Part model, mm, in its own coordinate system. Coordinates: 2 decimals unless noted, no trailing zeros. Loops run counter-clockwise (first coordinate to the right, second up) from the corner with the lowest first, then second, coordinate; pieces in that order, holes last. Notation, with made-up numbers: (68, 73.25) - (86, 73.25) arc R19 cw to (86, 89.25) - close; hole circle Ø7 at (48, 31). An arc over 180 degrees is marked (long way). Use a Markdown table: item, result. Add a question column.
1. Drop flat-ended pins along their axis: pin 1 (1 mm diameter, centred on x = -13.5, y = 1, fed in from -Z); pin 2 (1.2 mm diameter, centred on y = 2, z = 21.5, fed in from +X); pin 3 (1.2 mm diameter, centred on y = 1.5, z = -75, fed in from +X); pin 4 (4 mm diameter, centred on x = 23, z = 2, fed in from -Y). Give the stop position or say it passes through.
2. Band-saw the part on C-C, the plane z = 27.5. Give the cut face in (x, y), plus the area to 3 significant figures.
3. Wall check: probe 1 along Z at (x, y) = (44.5, 2.1); probe 2 along Z at (x, y) = (-73.5, 1.25); probe 3 along X at (y, z) = (2.3, -14.5). Give the ranges that are in metal, low to high. Write a range as [from, to].
4. Band-saw the part on B-B, the plane y = 2.1. Count the separate pieces of the cut face and the enclosed holes in it, plus the area to 4 significant figures.
5. Band-saw the part on A-A, the plane x = 134. Give the cut face in (y, z), plus the area to 3 significant figures.
from build123d import *

# Parameters (mm, degrees)
SKETCH1_2_W         = 20
SKETCH1_2_H         = 2.5
BOSS_EXTRUDE2_DEPTH = 2.5


with BuildPart() as part:
    # Sketch1_2 → Boss-Extrude2 (new body)
    with BuildSketch(Plane(origin=(0, 0, 0), x_dir=(1, 0, 0), z_dir=(0, 1, 0))):
        Polygon((-180, -72.5), (-180, -77.5), (-160, -77.5), (-160, -72.5), (-137.5, -72.5), (-137.5, -77.5), (-117.5, -77.5), (-117.5, -72.5), (-95, -72.5), (-95, -77.5), (-75, -77.5), (-75, -72.5), (-52.5, -72.5), (-52.5, -77.5), (-32.5, -77.5), (-32.5, -72.5), (-10, -72.5), (-10, -77.5), (10, -77.5), (10, -72.5), (32.5, -72.5), (32.5, -77.5), (52.5, -77.5), (52.5, -72.5), (75, -72.5), (75, -77.5), (95, -77.5), (95, -72.5), (117.5, -72.5), (117.5, -77.5), (137.5, -77.5), (137.5, -72.5), (160, -72.5), (160, -77.5), (180, -77.5), (180, -72.5), (190, -72.5), (190, -57.5), (195, -57.5), (195, -37.5), (190, -37.5), (190, -10), (195, -10), (195, 10), (190, 10), (190, 37.5), (195, 37.5), (195, 57.5), (190, 57.5), (190, 72.5), (180, 72.5), (180, 77.5), (160, 77.5), (160, 72.5), (137.5, 72.5), (137.5, 77.5), (117.5, 77.5), (117.5, 72.5), (95, 72.5), (95, 77.5), (75, 77.5), (75, 72.5), (52.5, 72.5), (52.5, 77.5), (32.5, 77.5), (32.5, 72.5), (10, 72.5), (10, 77.5), (-10, 77.5), (-10, 72.5), (-32.5, 72.5), (-32.5, 77.5), (-52.5, 77.5), (-52.5, 72.5), (-75, 72.5), (-75, 77.5), (-95, 77.5), (-95, 72.5), (-117.5, 72.5), (-117.5, 77.5), (-137.5, 77.5), (-137.5, 72.5), (-160, 72.5), (-160, 77.5), (-180, 77.5), (-180, 72.5), (-190, 72.5), (-190, 57.5), (-195, 57.5), (-195, 37.5), (-190, 37.5), (-190, 10), (-195, 10), (-195, -10), (-190, -10), (-190, -37.5), (-195, -37.5), (-195, -57.5), (-190, -57.5), (-190, -72.5), align=None)
        with Locations((-127.5, -21.25)):
            Rectangle(SKETCH1_2_W, SKETCH1_2_H, mode=Mode.SUBTRACT)
        with Locations((-170, -21.25)):
            Rectangle(SKETCH1_2_W, SKETCH1_2_H, mode=Mode.SUBTRACT)
        with Locations((-85, -21.25)):
            Rectangle(SKETCH1_2_W, SKETCH1_2_H, mode=Mode.SUBTRACT)
        with Locations((-42.5, -21.25)):
            Rectangle(SKETCH1_2_W, SKETCH1_2_H, mode=Mode.SUBTRACT)
        with Locations((0, -21.25)):
            Rectangle(SKETCH1_2_W, SKETCH1_2_H, mode=Mode.SUBTRACT)
        with Locations((42.5, -21.25)):
            Rectangle(SKETCH1_2_W, SKETCH1_2_H, mode=Mode.SUBTRACT)
        with Locations((85, -21.25)):
            Rectangle(SKETCH1_2_W, SKETCH1_2_H, mode=Mode.SUBTRACT)
        with Locations((127.5, -21.25)):
            Rectangle(SKETCH1_2_W, SKETCH1_2_H, mode=Mode.SUBTRACT)
        with Locations((170, -21.25)):
            Rectangle(SKETCH1_2_W, SKETCH1_2_H, mode=Mode.SUBTRACT)
    extrude(amount=BOSS_EXTRUDE2_DEPTH)


solid = part.part
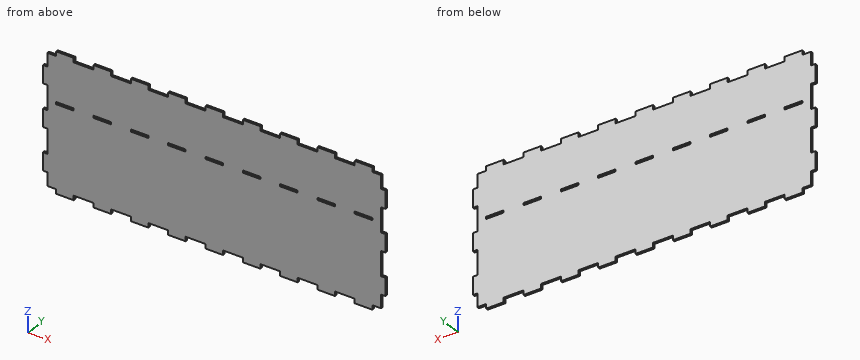
Geometry check:
| question | item | result |
|---|---|---|
| 1 | pin 1 | stops at z = -72.5 |
| 1 | pin 2 | stops at x = 190 |
| 1 | pin 3 | stops at x = 180 |
| 1 | pin 4 | stops at y = 0 |
| 2 | outline | (-190, 0) - (190, 0) - (190, 2.5) - (-190, 2.5) - close |
| 2 | area | 950 mm^2 |
| 3 | probe 1 | z = [-77.5, 20], [22.5, 77.5] |
| 3 | probe 2 | z = [-72.5, 72.5] |
| 3 | probe 3 | x = [-190, 190] |
| 4 | separate pieces | 1 |
| 4 | enclosed holes | 9 |
| 4 | area | 57,050 mm^2 |
| 5 | outline | (0, -77.5) - (2.5, -77.5) - (2.5, 20) - (0, 20) - close; (0, 22.5) - (2.5, 22.5) - (2.5, 77.5) - (0, 77.5) - close |
| 5 | area | 381 mm^2 |
